```python
from build123d import *

# Parameters (mm, degrees)
F0_R     = 47.5
F0_R_2   = 41
F1_DEPTH = 5
F2_R     = 50
F2_R_2   = 47
F3_DEPTH = 21
F4_R     = 5
F5_SIZE  = 2


with BuildPart() as f1:
    # F0 (on Top) → F1 (new body)
    with BuildSketch(Plane.XY):
        Circle(F0_R)
        Circle(F0_R_2, mode=Mode.SUBTRACT)
    extrude(amount=F1_DEPTH)

    # F2 (on Top) → F3 (join)
    with BuildSketch(Plane.XY):
        Circle(F2_R)
        Circle(F2_R_2, mode=Mode.SUBTRACT)
    extrude(amount=F3_DEPTH)

    # F4
    f4_edges = [f1.edges().sort_by_distance(p)[0] for p in [
        (-50, 0, 0),
    ]]
    fillet(f4_edges, radius=F4_R)

    # F5
    f5_edges = [f1.edges().sort_by_distance(p)[0] for p in [
        (-50, 0, 21),
    ]]
    chamfer(f5_edges, length=F5_SIZE)


solid = f1.part
```
Design review of the part built by this model. Coordinates are the model's own, in mm. A direction names the side the tool comes from. Give positions to 0.01 mm unless a question says otherwise; leave off trailing zeros. Order: outer loops, then holes, each group sorted by start corner. A loop starts at its lowest first (then second) coordinate and runs counter-clockwise, first axis right, second up. Notation, with made-up numbers: (59, -28) -> (75, -28) arc R26 cw to (75, -11) -> close; hole circle Ø11 at (65, 36). An arc over 180 degrees is marked (long way). Write item = value, one per line. Start each with the question number.
(1) For faces 1 (the face through (35, -32, 21)), 2 (the face through (-14, 39, 5)), list the 3-axis set-ups (+Z, -Z, +X, -X, +Y, -Y) from which the entire face can be reached by the end or side of a thin tool; tool diameter is ignored.
(2) Mouldability with a two-part tool opening along Y and no side actions: class faces 3 (the face through (44.83, 14.12, 12.89)), 4 (the face through (47.69, 15.02, 11.9)), 5 (the face through (-10, -40, 0)) as +Y half, -Y half, draft (parallel to the pull), parting line (faces both ways), or undercut.
(3) We need section A-A on x = 0. Write out the cut boundary in (y, z), plus the area to 3 significant figures.
(4) We need section D-D on z = 2. Write out the cut boundary in (x, y).
(5) For pin 1 (2 mm diameter, centred on y = -35.5, z = 2.5, fed in from +X); pin 2 (1 mm diameter, centred on y = 26.5, z = 7.5, fed in from +X); pin 3 (5 mm diameter, centred on x = -31, y = -29.5, fed in from +Z), all flat-tipped, find the tip position at first contact; note any pin that passes through.
(6) We need section C-C on z = 8. Write out the cut boundary in (x, y), plus the area to 3 significant figures.
(7) To check wall thickness, follow line 1 along Y through (x, z) = (-1.5, 7.75); line 2 along Z through (x, y) = (41, 12); line 3 along Y through (x, z) = (33, 9.75). State the ranges of each line that lie inside material, in increasing order.
Numbers:
q1.face_1 = +Z, +X, -X, +Y, -Y
q1.face_2 = +Z
q2.face_3 = undercut
q2.face_4 = parting line
q2.face_5 = draft
q3.outline = (-50, 5) arc R5 ccw to (-45, 0) -> (-41, 0) -> (-41, 5) -> (-47, 5) -> (-47, 21) -> (-48, 21) -> (-50, 19) -> close; (41, 0) -> (45, 0) arc R5 ccw to (50, 5) -> (50, 19) -> (48, 21) -> (47, 21) -> (47, 5) -> (41, 5) -> close
q3.area = 171 mm^2
q4.outline = circle Ø98 at (0, 0); hole circle Ø82 at (0, 0)
q5.pin_1 = 35.48
q5.pin_2 = 42.71
q5.pin_3 = 5
q6.outline = circle Ø100 at (0, 0); hole circle Ø94 at (0, 0)
q6.area = 914 mm^2
q7.line_1 = -49.98 to -46.98, 46.98 to 49.98
q7.line_2 = 0 to 5
q7.line_3 = -37.56 to -33.47, 33.47 to 37.56
